from build123d import *

# Parameters (mm, degrees)
F1_DEPTH = 25
F0_W     = 20
F0_H     = 11
F2_DEPTH = 7.5
F3_DEPTH = 2.5
F5_R     = 5


with BuildPart() as f1:
    # F0 (on Front) → F1 (new body, symmetric)
    with BuildSketch(Plane.XZ):
        Polygon((-25, -4), (25, -4), (25, 4), (14, 4), (-25, 4), align=None)
    extrude(amount=F1_DEPTH, both=True)

    # F0 (on Front) → F2 (join, symmetric)
    with BuildSketch(Plane.XZ):
        with BuildLine():
            Line((14, 4), (25, 4))
            Line((25, 4), (25, 11))
            ThreePointArc((25, 11), (26.4644660941, 14.5355339059), (30, 16))
            Line((30, 16), (32, 16))
            Line((32, 16), (32, 27))
            Line((32, 27), (30, 27))
            add(Edge.make_bspline(
                [(29.6159675373, 26.9953905569), (29.7437702017, 26.9970094957), (29.8717809107, 26.9985454717), (30, 27)],
                knots=[0.995223957, 0.995223957, 0.995223957, 0.995223957, 1, 1, 1, 1], degree=3))
            ThreePointArc((29.6159675373, 26.9953905569), (18.5513206132, 22.1771078682), (14, 11))
            Line((14, 11), (14, 4))
        make_face()
        with Locations((42, 21.5)):
            Rectangle(F0_W, F0_H)
    extrude(amount=F2_DEPTH, both=True)

    # F0 (on Front) → F3 (join, symmetric)
    with BuildSketch(Plane.XZ):
        with BuildLine():
            add(Edge.make_bspline(
                [(-25, 4), (-20.9363555228, 11.1345288275), (-6.6078681518, 24.5104887957), (15.0992011527, 26.8114995805), (29.6159675373, 26.9953905569)],
                knots=[0, 0, 0, 0, 0.4527258751, 0.995223957, 0.995223957, 0.995223957, 0.995223957], degree=3))
            Line((-25, 4), (14, 4))
            Line((14, 4), (14, 11))
            ThreePointArc((14, 11), (18.5513206132, 22.1771078682), (29.6159675373, 26.9953905569))
        make_face()
    extrude(amount=F3_DEPTH, both=True)

    # F0 (on Front) → F4 (revolve)
    with BuildSketch(Plane.XZ):
        Polygon((52, 27), (52, 16), (52, 14), (72, 14), (72, 29), (52, 29), align=None)
    revolve(axis=Axis((52, 0, 21.5), (0, 0, 1)))

    # F5
    f5_edges = [f1.edges().sort_by_distance(p)[0] for p in [
        (25, 25, 0),
        (-25, 25, 0),
        (-25, -25, 0),
        (25, -25, 0),
    ]]
    fillet(f5_edges, radius=F5_R)


solid = f1.part
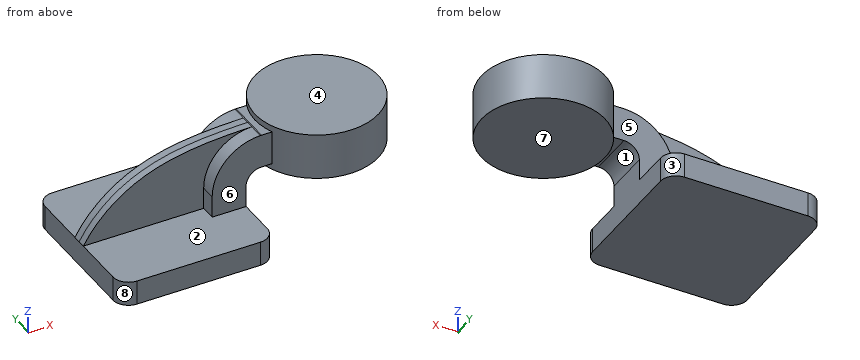
Geometry check sheet. Reference: the model listing, model coordinates, mm. Face numbers are marked on the shaded views. A direction names the side the tool comes from. Round coordinates to 2 decimals unless told otherwise and drop trailing zeros. Loops run counter-clockwise (first coordinate to the right, second up) from the corner with the lowest first, then second, coordinate; pieces in that order, holes last. Notation, with made-up numbers: (23.5, 43.25) -> (58.5, 43.25) arc R8 cw to (58.5, 58.25) -> close; hole circle Ø1 at (-23.5, -20.75). An arc over 180 degrees is marked (long way). Answer as a JSON object with one key per item and string values. Group by question number.
Item 1: Set-up check for the marked faces 4, 5, 6, 7 and 8: record each of +Z, -Z, +X, -X, +Y, -Y from which the full face is reachable in a straight line by a thin tool's end or side.
Item 2: Cross-section at C-C, the plane x = 42. Record the cut outline in (y, z), plus the area to 3 significant figures.
Item 3: Cross-section at A-A, the plane y = 16.5. Record the cut outline in (x, z).
Item 4: Thickness scan on line 1 along Z through (x, y) = (19.5, -10.5); line 2 along Y through (x, z) = (3.5, 17); line 3 along Z through (x, y) = (55.5, -1). Record the ranges inside material, lowest first.
Item 5: Cross-section at B-B, the plane x = 52. Record the cut outline in (y, z).
Item 6: Depth check by flat-ended pin: pin 1 Ø12 at (x, y) = (60, -3.5) entering from -Z; pin 2 Ø9.5 at (x, z) = (24, 15) entering from -Y; pin 3 Ø1.5 at (y, z) = (-4, 7) entering from -X. Enter the tip coordinate at first touch or a pass-through.
Item 7: Release check for a two-part mould opening along X. For the marked faces 1, 2 and 3 record: pulls with the +X half, pulls with the -X half, needs draft (parallel to the pull), parting line crosses it, or undercut.
Determined:
{
 "1": {"face 4": "+Z, +X, -X, +Y, -Y", "face 5": "+Z, -X, +Y", "face 6": "+Z, -X, -Y", "face 7": "-Z, +X, +Y, -Y", "face 8": "+Z, -Z, -X, -Y"},
 "2": {"outline": "(-17.32, 14) -> (17.32, 14) -> (17.32, 29) -> (-17.32, 29) -> close", "area": "520 mm²"},
 "3": {"outline": "(-25, -4) -> (25, -4) -> (25, 4) -> (-25, 4) -> close; (40.7, 14) -> (63.3, 14) -> (63.3, 29) -> (40.7, 29) -> close"},
 "4": {"line 1": "z = -4 to 4", "line 2": "y = -2.5 to 2.5", "line 3": "z = 14 to 29"},
 "5": {"outline": "(-20, 14) -> (20, 14) -> (20, 29) -> (-20, 29) -> close"},
 "6": {"pin 1": "stops at z = 14", "pin 2": "stops at y = -7.5", "pin 3": "stops at x = 14"},
 "7": {"face 1": "undercut", "face 2": "needs draft", "face 3": "pulls with the +X half"}
}
